```python
from build123d import *

# Parameters (mm, degrees)
SKETCH1_R                           = 22.5
SKETCH1_R_2                         = 12.5
BOSS_EXTRUDE1_DEPTH                 = 10
M5_CLEARANCE_HOLE1_D                = 5.3
F_3_0MM_CLEARANCE_DOWEL_HOLE1_D     = 3.016
F_3_0MM_CLEARANCE_DOWEL_HOLE1_DEPTH = 5
F_3_0MM_CLEARANCE_DOWEL_HOLE1_TIP   = 0.906097813
F_2_9_2_9_DIAMETER_HOLE1_D          = 2.9
F_2_9_2_9_DIAMETER_HOLE1_DEPTH      = 7
F_2_9_2_9_DIAMETER_HOLE1_TIP        = 0.871247898
CUT_EXTRUDE1_START                  = -5.906098
CUT_EXTRUDE1_DEPTH                  = 5.906098
CHAMFER1_SIZE                       = 1
CHAMFER2_SIZE                       = 0.181985117
CHAMFER2_SIZE_2                     = 0.5


with BuildPart() as part:
    # Sketch1 → Boss-Extrude1 (new, symmetric)
    with BuildSketch(Plane.XY):
        Circle(SKETCH1_R)
        Circle(SKETCH1_R_2, mode=Mode.SUBTRACT)
    extrude(amount=BOSS_EXTRUDE1_DEPTH, both=True)

    # M5 Clearance Hole1 (through all)
    with Locations(Plane.XY.offset(10)):
        with Locations((6.696960066, -16.167891819), (16.167891819, -6.696960066), (16.167891819, 6.696960066), (6.696960066, 16.167891819), (-6.696960066, 16.167891819), (-16.167891819, 6.696960066), (-16.167891819, -6.696960066), (-6.696960066, -16.167891819)):
            Hole(M5_CLEARANCE_HOLE1_D / 2)

    # Ø3.0mm Clearance Dowel Hole1
    with Locations(Plane.XY.offset(10)):
        with Locations((-17.5, 0), (17.5, 0)):
            Hole(F_3_0MM_CLEARANCE_DOWEL_HOLE1_D / 2, depth=F_3_0MM_CLEARANCE_DOWEL_HOLE1_DEPTH)
            with Locations((0, 0, -(F_3_0MM_CLEARANCE_DOWEL_HOLE1_DEPTH + F_3_0MM_CLEARANCE_DOWEL_HOLE1_TIP / 2))):  # 118° drill point
                Cone(0, F_3_0MM_CLEARANCE_DOWEL_HOLE1_D / 2, F_3_0MM_CLEARANCE_DOWEL_HOLE1_TIP, mode=Mode.SUBTRACT)

    # Ø2.9 (2.9) Diameter Hole1
    with Locations(Plane(origin=(0, 0, -10), x_dir=(-1, 0, 0), z_dir=(0, 0, -1))):
        with Locations((-17.5, 0), (17.5, 0)):
            Hole(F_2_9_2_9_DIAMETER_HOLE1_D / 2, depth=F_2_9_2_9_DIAMETER_HOLE1_DEPTH)
            with Locations((0, 0, -(F_2_9_2_9_DIAMETER_HOLE1_DEPTH + F_2_9_2_9_DIAMETER_HOLE1_TIP / 2))):  # 118° drill point
                Cone(0, F_2_9_2_9_DIAMETER_HOLE1_D / 2, F_2_9_2_9_DIAMETER_HOLE1_TIP, mode=Mode.SUBTRACT)

    # Sketch8 → Cut-Extrude1 (cut)
    with BuildSketch(Plane.XY.offset(10).offset(CUT_EXTRUDE1_START)):
        with BuildLine():
            Line((17.25, 1.508), (17.75, 1.508))
            ThreePointArc((17.75, 1.508), (19.258, 0), (17.75, -1.508))
            Line((17.75, -1.508), (17.25, -1.508))
            ThreePointArc((17.25, -1.508), (15.742, 0), (17.25, 1.508))
        make_face()
    extrude(amount=CUT_EXTRUDE1_DEPTH, mode=Mode.SUBTRACT)

    # Chamfer1
    chamfer1_edges = [part.edges().sort_by_distance(p)[0] for p in [
        (-22.5, 0, -10),
        (-22.5, 0, 10),
        (-12.5, 0, -10),
        (-12.5, 0, 10),
    ]]
    chamfer(chamfer1_edges, length=CHAMFER1_SIZE)

    # Chamfer2
    # the kernel refuses this chamfer: 0.5, 0.181985117 mm, written as the material it takes off along each edge
    with BuildSketch(Plane(origin=(-17.5, 0, 10), x_dir=(-1, 0, 0), z_dir=(0, -1, 0))) as chamfer2_piece_1:
        Polygon((1.508 + CHAMFER2_SIZE, 0), (1.508, CHAMFER2_SIZE_2), (1.508, 0), align=None)
    revolve(axis=Axis((-17.5, 0, 10), (0, 0, -1)), mode=Mode.SUBTRACT)
    with BuildSketch(Plane(origin=(-17.5, 0, -10), x_dir=(1, 0, 0), z_dir=(0, -1, 0))) as chamfer2_piece_2:
        Polygon((1.45 + CHAMFER2_SIZE, 0), (1.45, CHAMFER2_SIZE_2), (1.45, 0), align=None)
    revolve(axis=Axis((-17.5, 0, -10), (0, 0, 1)), mode=Mode.SUBTRACT)
    with BuildSketch(Plane(origin=(17.5, 0, -10), x_dir=(1, 0, 0), z_dir=(0, -1, 0))) as chamfer2_piece_3:
        Polygon((1.45 + CHAMFER2_SIZE, 0), (1.45, CHAMFER2_SIZE_2), (1.45, 0), align=None)
    revolve(axis=Axis((17.5, 0, -10), (0, 0, 1)), mode=Mode.SUBTRACT)
    with BuildSketch(Plane(origin=(17.75, -1.508, 10), x_dir=(0, -0.9950833631817482, 0.09904090225205342), z_dir=(-1, 0, 0)), Plane(origin=(17.5, 1.508, 10), x_dir=(0, 0.9950833631817482, 0.09904090225205342), z_dir=(1, 0, 0)), Plane(origin=(17.5, -1.508, 10), x_dir=(0, -0.9950833631817482, 0.09904090225205342), z_dir=(-1, 0, 0)), Plane(origin=(17.25, 1.508, 10), x_dir=(0, 0.9950833631817482, 0.09904090225205342), z_dir=(1, 0, 0))) as chamfer2_piece_4:
        Polygon((CHAMFER2_SIZE * 0.99508336391, -CHAMFER2_SIZE * 0.0990409023245), (-CHAMFER2_SIZE_2 * 0.0990409022521, -CHAMFER2_SIZE_2 * 0.995083363182), (0, 0), align=None)
    extrude(amount=0.25, mode=Mode.SUBTRACT)
    with BuildSketch(Plane(origin=(17.25, 0, 10), x_dir=(0, -1, 0), z_dir=(1, 0, 0))) as chamfer2_piece_5:
        Polygon((1.508 + CHAMFER2_SIZE, 0), (1.508, CHAMFER2_SIZE_2), (1.508, 0), align=None)
    revolve(axis=Axis((17.25, 0, 10), (0, 0, -1)), revolution_arc=180, mode=Mode.SUBTRACT)
    with BuildSketch(Plane(origin=(17.75, 0, 10), x_dir=(0, 1, 0), z_dir=(-1, 0, 0))) as chamfer2_piece_6:
        Polygon((1.508 + CHAMFER2_SIZE, 0), (1.508, CHAMFER2_SIZE_2), (1.508, 0), align=None)
    revolve(axis=Axis((17.75, 0, 10), (0, 0, -1)), revolution_arc=180, mode=Mode.SUBTRACT)


solid = part.part
```
Geometry check sheet. Reference: the model listing, model coordinates, mm. A direction names the side the tool comes from. Give positions to 0.01 mm unless a question says otherwise; leave off trailing zeros. Order: outer loops, then holes, each group sorted by start corner. A loop starts at its lowest first (then second) coordinate and runs counter-clockwise, first axis right, second up.
1. Access from +Z, -Z, +X, -X, +Y, -Y to the whole of each face (thin tool, end or side, straight path). Record for faces 1 (the face through (-16.12, 0.44, -6.2)), 2 (the face through (19.258, 0.033, 6.759)), 3 (the face through (8.8, 14.555, -0.14)).
2. Release check for a two-part mould opening along X. For faces 4 (the face through (15.673, -0.035, 9.691)), 5 (the face through (0, -14, 10)) record: pulls with the +X half, pulls with the -X half, needs draft (parallel to the pull), parting line crosses it, or undercut.
3. Thickness scan on L1, parallel to Y at x = 17, z = 2.75; L2, parallel to X at y = -5, z = -7.25. Record the ranges inside material, lowest first.
4. Section check A-A, the plane x = 0. Enter the section's corners in (y, z), and give its area (3 significant figures).
5. Gauge pin test, flat ends, axial feed: pin 1 Ø5 at (x, y) = (-16.17, -6.7) entering from -Z; pin 2 Ø1.5 at (y, z) = (3.5, 2) entering from -X; pin 3 Ø8 at (y, z) = (-6.5, 3.5) entering from -X; pin 4 Ø6 at (x, z) = (0, -7.5) entering from +Y. Record the tip position at first contact, or that the pin passes through.
6. Section check B-B, the plane z = -8.25. Give the number of separate pieces and of enclosed holes in the cut face, and give its area (3 significant figures).
Values follow:
1. face 1: -Z
1. face 2: +Z
1. face 3: +Z, -Z
2. face 4: undercut
2. face 5: needs draft
3. L1: y = -14.74 to -9.21, -4.18 to 4.18, 9.21 to 14.74
3. L2: x = -21.94 to -18.2, -14.13 to -11.46, 11.46 to 14.13, 18.2 to 21.94
4. outline: (-22.5, -9) - (-21.5, -10) - (-13.5, -10) - (-12.5, -9) - (-12.5, 9) - (-13.5, 10) - (-21.5, 10) - (-22.5, 9) - close; (12.5, -9) - (13.5, -10) - (21.5, -10) - (22.5, -9) - (22.5, 9) - (21.5, 10) - (13.5, 10) - (12.5, 9) - close
4. area: 396 mm2
5. pin 1: passes through
5. pin 2: stops at x = -22.33
5. pin 3: stops at x = -22.36
5. pin 4: stops at y = 22.5
6. separate pieces: 1
6. enclosed holes: 11
6. area: 910 mm2
